The drawing under review shows one solid part. Ordinate dimensions are in mm from its lowest x, y, z. Coordinates: 2 decimals unless noted, no trailing zeros. Order: outer loops, then holes, each group sorted by start corner. A loop starts at its lowest first (then second) coordinate and runs counter-clockwise, first axis right, second up.
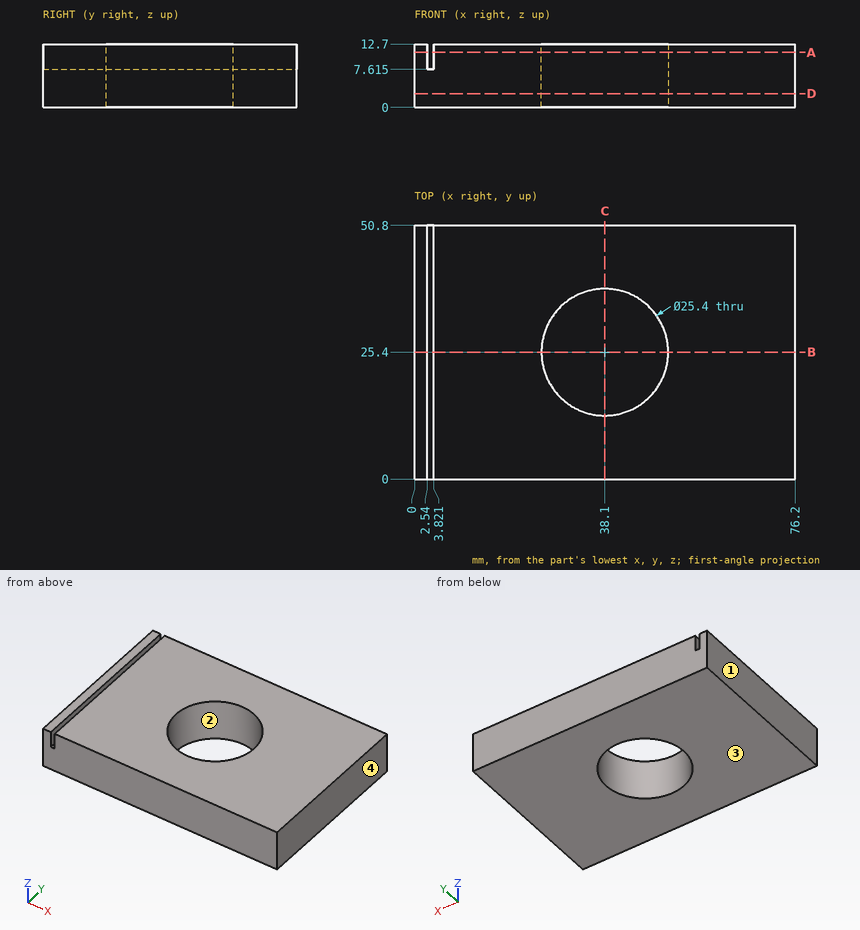
1. Add section B-B (y = 25.4). Give the boundary of the cut face in (x, z) (1 decimal).
2. Add section A-A (z = 11). Give the boundary of the cut face in (x, y), and give its area (3 significant figures).
3. Mouldability with a two-part tool opening along X and no side actions: class the marked faces 1, 2, 3 and 4 as pulls with the +X half, pulls with the -X half, needs draft (parallel to the pull), parting line crosses it, or undercut.
4. Add section C-C (x = 38.1). Give the boundary of the cut face in (y, z).
5. Add section D-D (z = 2.75). Give the boundary of the cut face in (x, y).
6. To check wall thickness, follow line 1 (X direction, y = 25, z = 9.5); line 2 (Y direction, x = 38.1, z = 6); line 3 (X direction, y = 8, z = 10.5). State the ranges of each line that lie inside material, in increasing order.
Solution:
1. outline: (0, 0) - (25.4, 0) - (25.4, 12.7) - (3.8, 12.7) - (3.8, 7.6) - (2.5, 7.6) - (2.5, 12.7) - (0, 12.7) - close; (50.8, 0) - (76.2, 0) - (76.2, 12.7) - (50.8, 12.7) - close
2. outline: (0, 0) - (2.54, 0) - (2.54, 50.8) - (0, 50.8) - close; (3.82, 0) - (76.2, 0) - (76.2, 50.8) - (3.82, 50.8) - close; hole circle Ø25.4 at (38.1, 25.4)
2. area: 3,300 mm2
3. face 1: pulls with the -X half
3. face 2: undercut
3. face 3: needs draft
3. face 4: pulls with the +X half
4. outline: (0, 0) - (12.7, 0) - (12.7, 12.7) - (0, 12.7) - close; (38.1, 0) - (50.8, 0) - (50.8, 12.7) - (38.1, 12.7) - close
5. outline: (0, 0) - (76.2, 0) - (76.2, 50.8) - (0, 50.8) - close; hole circle Ø25.4 at (38.1, 25.4)
6. line 1: x = 0 to 2.54, 3.82 to 25.41, 50.79 to 76.2
6. line 2: y = 0 to 12.7, 38.1 to 50.8
6. line 3: x = 0 to 2.54, 3.82 to 76.2
